Design review of the part shown in the three views and the two pictorial views. Dimensions are in mm from the part's minimum x, y and z. Give positions to 0.01 mm unless a question says otherwise; leave off trailing zeros. Loops run counter-clockwise (first coordinate to the right, second up) from the corner with the lowest first, then second, coordinate; pieces in that order, holes last. Notation, with made-up numbers: (7, 33.5) -> (44, 33.5) arc R19 ccw to (44, 45.5) -> close; hole circle Ø5 at (-2.75, -9.75). An arc over 180 degrees is marked (long way). Answer as CSV lines item,"result". Start each with the question number.
Item 1: For L1, parallel to X at y = 152, z = 1.75; L2, parallel to X at y = 272, z = 2.9; L3, parallel to X at y = 246, z = 0.9, list the stretches that pass through material, from the lowest coordinate up. Write a range as from..to.
Item 2: Add section D-D on x = 24. State the section outline as (y, z) points.
Item 3: Clearance check with flat-ended pins moving along their axes: P1, Ø1.5, axis at x = 39.5, y = 181, coming from the -Z side; P2, Ø1.8, axis at x = 252, z = 4, coming from the +Y side; P3, Ø3, axis at x = 252.5, z = 2.5, coming from the -Y side; P4, Ø1.8, axis at x = 288, z = 4.5, coming from the -Y side. State where each tip first meets the part, or that it passes through.
Item 4: Add section C-C on y = 38. State the section outline as (x, z) points, plus the area to 3 significant figures.
Item 5: Add section B-B on z = 2.4. State the section outline as (x, y) points.
Item 6: Add section A-A on x = 255. State the section outline as (y, z) points, plus the area to 3 significant figures.
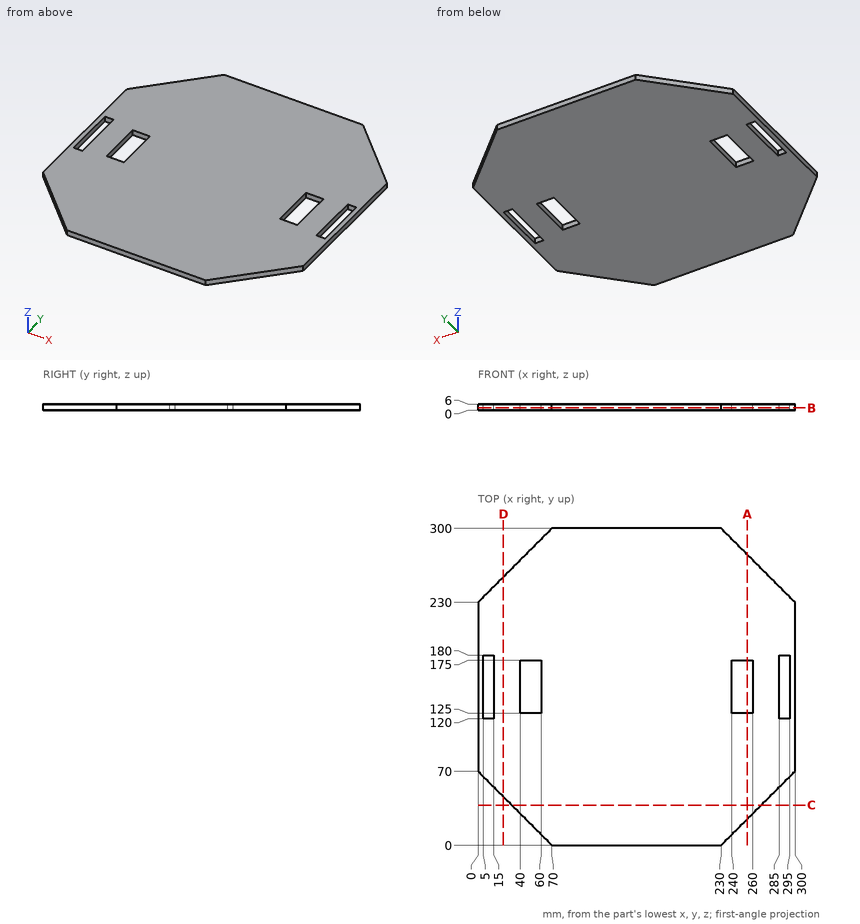
Computed values:
1,L1,"0..5, 15..40, 60..240, 260..285, 295..300"
1,L2,"42..258"
1,L3,"16..284"
2,outline,"(46, 0) -> (254, 0) -> (254, 6) -> (46, 6) -> close"
3,P1,"z = 0"
3,P2,"y = 278.9"
3,P3,"y = 21"
3,P4,"y = 57.1"
4,outline,"(32, 0) -> (268, 0) -> (268, 6) -> (32, 6) -> close"
4,area,"1,420 mm²"
5,outline,"(0, 70) -> (70, 0) -> (230, 0) -> (300, 70) -> (300, 230) -> (230, 300) -> (70, 300) -> (0, 230) -> close; hole (5, 120) -> (15, 120) -> (15, 180) -> (5, 180) -> close; hole (40, 125) -> (60, 125) -> (60, 175) -> (40, 175) -> close; hole (240, 125) -> (260, 125) -> (260, 175) -> (240, 175) -> close; hole (285, 120) -> (295, 120) -> (295, 180) -> (285, 180) -> close"
6,outline,"(25, 0) -> (125, 0) -> (125, 6) -> (25, 6) -> close; (175, 0) -> (275, 0) -> (275, 6) -> (175, 6) -> close"
6,area,"1,200 mm²"
